from build123d import *

# Parameters (mm, degrees)
BOSS_EXTRUDE1_DEPTH     = 72
SKETCH2_W               = 48
SKETCH2_H               = 20
BOSS_EXTRUDE2_DEPTH     = 120
CUT_EXTRUDE1_DEPTH      = 121.066648158
CUT_EXTRUDE1_DEPTH_BACK = 121.066648158
SKETCH4_R               = 24
SKETCH5_W               = 64
SKETCH5_H               = 20
BOSS_EXTRUDE3_DEPTH     = 48
CUT_EXTRUDE2_DEPTH      = 136.823414771
CUT_EXTRUDE2_DEPTH_BACK = 136.823414771
SKETCH6_R               = 8


with BuildPart() as part:
    # Sketch1 → Boss-Extrude1 (new, symmetric)
    with BuildSketch(Plane.YZ):
        with BuildLine():
            Line((-40, 0), (-24, 0))
            ThreePointArc((-24, 0), (0, -24), (24, 0))
            Line((24, 0), (40, 0))
            ThreePointArc((40, 0), (0, -40), (-40, 0))
        make_face()
    extrude(amount=BOSS_EXTRUDE1_DEPTH, both=True)

    # Sketch2 → Boss-Extrude2 (add)
    with BuildSketch(Plane(origin=(0, 60, 0), x_dir=(-1, 0, 0), z_dir=(0, 1, 0))):
        with Locations((0, -10)):
            Rectangle(SKETCH2_W, SKETCH2_H)
    extrude(amount=-BOSS_EXTRUDE2_DEPTH)

    # Sketch4 → Cut-Extrude1 (cut, two sides: drawn at the far end of the back side and taken through both)
    with BuildSketch(Plane.YZ.offset(24).offset(-CUT_EXTRUDE1_DEPTH_BACK)):
        Circle(SKETCH4_R)
    extrude(amount=CUT_EXTRUDE1_DEPTH + CUT_EXTRUDE1_DEPTH_BACK, mode=Mode.SUBTRACT)

    # Sketch5 → Boss-Extrude3 (add)
    with BuildSketch(Plane(origin=(0, 60, 0), x_dir=(-1, 0, 0), z_dir=(0, 1, 0))):
        with Locations((0, -20)):
            Rectangle(SKETCH5_W, SKETCH5_H)
    boss_extrude3 = extrude(amount=BOSS_EXTRUDE3_DEPTH)

    # Mirror1: Boss-Extrude3 across plane
    add(boss_extrude3.mirror(Plane.ZX))

    # Sketch6 → Cut-Extrude2 (cut, two sides: drawn at the far end of the back side and taken through both)
    with BuildSketch(Plane.XY.offset(-CUT_EXTRUDE2_DEPTH_BACK)):
        with Locations(Location((0, 40, 0), (0, 0, 317.942751882))):
            Circle(SKETCH6_R)
        with Locations(Location((0, -40, 0), (0, 0, 42.057262179))):
            Circle(SKETCH6_R)
        with BuildLine():
            Line((8, 92), (8, 76))
            ThreePointArc((8, 76), (0, 68), (-8, 76))
            Line((-8, 76), (-8, 92))
            ThreePointArc((-8, 92), (0, 100), (8, 92))
        make_face()
        with BuildLine():
            Line((8, -92), (8, -76))
            ThreePointArc((8, -76), (0, -68), (-8, -76))
            Line((-8, -76), (-8, -92))
            ThreePointArc((-8, -92), (0, -100), (8, -92))
        make_face()
    extrude(amount=CUT_EXTRUDE2_DEPTH + CUT_EXTRUDE2_DEPTH_BACK, mode=Mode.SUBTRACT)


solid = part.part
Can you work these out from the model? Positions are in its coordinate system, mm. A direction names the side the tool comes from. Coordinates: 2 decimals unless noted, no trailing zeros. Loops run counter-clockwise (first coordinate to the right, second up) from the corner with the lowest first, then second, coordinate; pieces in that order, holes last. Notation, with made-up numbers: M 21.5,78 L 51.5,78 A31 ccw 51.5,104 Z; hole C 58.5,84.25 d10. An arc over 180 degrees is marked long. Return JSON: item names as keys, results as strings. Group by question number.
Item 1: Imagine slicing it at D-D (x = -17.5). Please give me the cut outline in (y, z), and give its area (3 significant figures).
Item 2: Thinking about a two-plate mould opening in Y: for faces 5 (the flat face through (0, 108, -20)), 6 (the flat face through (-32, 84, -20)), 7 (the flat face through (0, -108, -20)), 8 (the flat face through (0, 60, -24)), which applies, released by +Y, released by -Y, zero draft, split by the parting line, or undercut?
Item 3: I'm going to push flat-ended pins straight in: pin 1 Ø6 at (y, z) = (-74.5, -23.5) entering from +X; pin 2 Ø14.5 at (x, y) = (-8.5, 76.5) entering from -Z; pin 3 Ø13 at (y, z) = (85.5, -17.5) entering from -X; pin 4 Ø6 at (x, y) = (35.5, 81) entering from -Z. Where does each tip first touch, or does it pass through?
Item 4: Imagine slicing it at B-B (y = 81). Please give me the cut outline in (x, z), and give its area (3 significant figures).
Item 5: On a 3-axis mill with a long thin cutter (end or side, diameter ignored), from which of +Z, -Z, +X, -X, +Y, -Y can I reach the whole of each face in a straight line? I mean faces 1 (the flat face through (0, -50, -20)), 2 (the flat face through (8, -73, -10)), 3 (the flat face through (32, -84, -20)), 4 (the flat face through (8, 73, -30)). Say none if no direction works.
Item 6: Imagine slicing it at C-C (z = -6.5). Please give me the cut outline in (x, y).
Item 7: If I drill on L1, parallel to X at y = -40, z = -16; L2, parallel to Y at x = 0, z = -11; L3, parallel to Y at x = 0, z = -5.5, over which ranges is the centre line in solid material (lowest first)? Write a range as from..to.
Item 8: Imagine slicing it at A-A (x = 0). Give the number of separate pieces and of enclosed holes in the cut face, and give its area (3 significant figures).
Verdict:
{
 "1": {"outline": "M -108,-30 L -60,-30 L -60,-20 L -34.64,-20 A40 ccw 34.64,-20 L 60,-20 L 60,-30 L 108,-30 L 108,-10 L 60,-10 L 60,0 L 24,0 A24 cw -24,0 L -60,0 L -60,-10 L -108,-10 Z", "area": "4,400 mm^2"},
 "2": {"face 5": "released by +Y", "face 6": "zero draft", "face 7": "released by -Y", "face 8": "undercut"},
 "3": {"pin 1": "stops at x = 32", "pin 2": "stops at z = -30", "pin 3": "stops at x = -32", "pin 4": "passes through"},
 "4": {"outline": "M -32,-30 L -8,-30 L -8,-10 L -32,-10 Z; M 8,-30 L 32,-30 L 32,-10 L 8,-10 Z", "area": "960 mm^2"},
 "5": {"face 1": "-Z, +X, -X", "face 2": "+Z, +X, -X, -Y", "face 3": "+Z, -Z, +X, -Y", "face 4": "-Z, +X, -X, +Y"},
 "6": {"outline": "M -72,-39.47 L -24,-39.47 L -24,-60 L 24,-60 L 24,-39.47 L 72,-39.47 L 72,-23.1 L -72,-23.1 Z; M -72,23.1 L 72,23.1 L 72,39.47 L 24,39.47 L 24,60 L -24,60 L -24,39.47 L -72,39.47 Z; hole C 0,-40 d16; hole C 0,40 d16"},
 "7": {"L1": "x = -24..-8, 8..24", "L2": "y = -108..-100, -68..-48, -32..-21.33, 21.33..32, 48..68, 100..108", "L3": "y = -60..-48, -32..-23.36, 23.36..32, 48..60"},
 "8": {"separate pieces": "5", "enclosed holes": "0", "area": "2,470 mm^2"}
}
